```python
from build123d import *

# Parameters (mm, degrees)
SKETCH_W         = 93.98
SKETCH_H         = 98.425
SKETCH_R         = 2.2225
PAD_DEPTH        = 8.89
SKETCH001_W      = 44.45
SKETCH001_H      = 74.93
POCKET_DEPTH     = 2.286
SKETCH002_R      = 3.4925
PAD001_DEPTH     = 6.147
POCKET001_DEPTH  = 98.426
CHAMFER_SIZE     = 3.81
CHAMFER001_SIZE2 = 77.1906
CHAMFER001_SIZE  = 19.0246
CHAMFER002_SIZE  = 2.54


with BuildPart() as part:
    # Sketch → Pad (new body)
    with BuildSketch(Plane.XY):
        with Locations((0, 49.2125)):
            Rectangle(SKETCH_W, SKETCH_H)
        with Locations((37.5, 86.811)):
            Circle(SKETCH_R, mode=Mode.SUBTRACT)
        with Locations((-37.5, 86.811)):
            Circle(SKETCH_R, mode=Mode.SUBTRACT)
        with Locations((-37.5, 11.811)):
            Circle(SKETCH_R, mode=Mode.SUBTRACT)
        with Locations((37.5, 11.811)):
            Circle(SKETCH_R, mode=Mode.SUBTRACT)
    extrude(amount=PAD_DEPTH)

    # Sketch001 → Pocket (cut)
    with BuildSketch(Plane.XY):
        with Locations((0, 37.465)):
            Rectangle(SKETCH001_W, SKETCH001_H)
    extrude(amount=POCKET_DEPTH, mode=Mode.SUBTRACT)

    # Sketch002 → Pad001 (join)
    with BuildSketch(Plane.XZ):
        Polygon((-19.05, 8.89), (-19.05, 27.94), (19.05, 27.94), (19.05, 8.89), (46.99, 8.89), (46.99, 0), (85.572552, 0), (66.7766, -28.194), (-70.5866, -28.194), (-45.863996, 8.89), align=None)
        with Locations((0, -10.1346)):
            Circle(SKETCH002_R, mode=Mode.SUBTRACT)
    extrude(amount=PAD001_DEPTH)

    # Sketch003 → Pocket001 (cut, through all)
    with BuildSketch(Plane.XZ):
        Polygon((-45.863996, 8.89), (-45.863996, 18.360811), (-55.502193, 18.360811), (-55.502193, -5.567332), align=None)
    extrude(amount=-POCKET001_DEPTH, mode=Mode.SUBTRACT)

    # Chamfer
    chamfer_edges = [part.edges().sort_by_distance(p)[0] for p in [
        (-70.5866, -3.0735, -28.194),
        (85.572552, -3.0735, 0),
    ]]
    chamfer(chamfer_edges, length=CHAMFER_SIZE)

    # Chamfer001
    chamfer001_edges = [part.edges().sort_by_distance(p)[0] for p in [
        (0, 0, 8.89),
    ]]
    chamfer001_side = part.faces().sort_by_distance((0, 0, 18.415))[0]
    chamfer(chamfer001_edges, length=CHAMFER001_SIZE, length2=CHAMFER001_SIZE2, reference=chamfer001_side)

    # Chamfer002
    chamfer002_edges = [part.edges().sort_by_distance(p)[0] for p in [
        (-19.05, 38.5953, 8.89),
        (-19.05, -3.0735, 8.89),
        (-46.99, 98.425, 3.600495),
        (46.99, 98.425, 4.445),
        (19.05, -3.0735, 8.89),
        (19.05, 38.5953, 8.89),
        (19.05, -3.0735, 27.94),
        (-19.05, -3.0735, 27.94),
        (46.99, 46.139, 8.89),
        (46.99, -3.0735, 0),
    ]]
    chamfer(chamfer002_edges, length=CHAMFER002_SIZE)


solid = part.part
```
Source: CAD feature listing. Evaluate the final solid. Frame: model axes, mm. A direction names the side the tool comes from. Round coordinates to 2 decimals unless told otherwise and drop trailing zeros. Loops run counter-clockwise (first coordinate to the right, second up) from the corner with the lowest first, then second, coordinate; pieces in that order, holes last. Notation, with made-up numbers: M 5.25,9 L 59.25,9 A19 cw 59.25,20 Z; hole C -26,71.25 d6. An arc over 180 degrees is marked long. Use a Markdown table: item, result. Add a question column.
1. Cut plane B-B, the plane x = 0. Output: boundary loops of the cut face in (y, z) (3 decimals).
2. Contact query for flat-ended pins moving along their axis: pin 1 (3 mm diameter, centred on y = 33.5, z = 16, fed in from +X); pin 2 (1 mm diameter, centred on x = -9, y = 50.5, fed in from +Z); pin 3 (7 mm diameter, centred on x = -37.5, y = 11.811, fed in from -Z); pin 4 (2.5 mm diameter, centred on x = -37.5, y = 86.811, fed in from +Z). Output: stop coordinate, or through.
3. Pull-direction query (X, two-part tool) for faces 6 (the flat face through (19.05, 23, 17)), 7 (the flat face through (9, -6.147, -6)), 8 (the cylindrical face through (-39.264, 10.459, 4.383)); classes: +X half, -X half, draft (parallel to the pull), parting line (faces both ways), or undercut.
4. Cut plane A-A, the plane x = -37.5. Output: boundary loops of the cut face in (y, z) (1 decimal).
5. Set-up query: faces 1 (the flat face through (65, -3, 0)), 2 (the flat face through (-1, 82, 8.89)), 3 (the flat face through (75.235, -3.03, -15.507)), 4 (the flat face through (0, 38, 2.286)), 5 (the flat face through (-19.05, 23, 17)). Return all of +Z, -Z, +X, -X, +Y, -Y with unobstructed straight access to the full face (end or side cutting, diameter ignored); none if empty.
6. Cut plane D-D, the plane x = 59. Output: boundary loops of the cut face in (y, z), and give its area (3 significant figures).
7. Ray query, line 1 along Y through (x, z) = (-37.5, 3.25) (1 decimal); line 2 along X through (y, z) = (13, 2) (3 decimals); line 3 along Z through (x, y) = (0, -1). Return the intervals inside material, ascending. Write a range as [from, to].
8. Cut plane C-C, the plane y = 43. Output: boundary loops of the cut face in (x, z) (3 decimals).
Solution:
| question | item | result |
|---|---|---|
| 1 | outline | M -6.147,-28.194 L 0,-28.194 L 0,-13.627 L -6.147,-13.627 Z; M -6.147,-6.642 L 0,-6.642 L 0,2.286 L 74.93,2.286 L 74.93,0 L 98.425,0 L 98.425,8.89 L 77.191,8.89 L 0,27.915 L 0,27.94 L -6.147,27.94 Z |
| 2 | pin 1 | stops at x = 19.05 |
| 2 | pin 2 | stops at z = 15.59 |
| 2 | pin 3 | stops at z = 0 |
| 2 | pin 4 | passes through |
| 3 | face 6 | +X half |
| 3 | face 7 | draft |
| 3 | face 8 | undercut |
| 4 | outline | M -6.1,-28.2 L 0,-28.2 L 0,0 L 9.6,0 L 9.6,8.9 L -6.1,8.9 Z; M 14,0 L 84.6,0 L 84.6,8.9 L 14,8.9 Z; M 89,0 L 98.4,0 L 98.4,8.9 L 89,8.9 Z |
| 5 | face 1 | +Z, +X, +Y, -Y |
| 5 | face 2 | +Z, +Y |
| 5 | face 3 | -Z, +X, +Y, -Y |
| 5 | face 4 | -Z |
| 5 | face 5 | +Z, -X, +Y, -Y |
| 6 | outline | M -6.15,-28.19 L 0,-28.19 L 0,0 L -6.15,0 Z |
| 6 | area | 173 mm2 |
| 7 | line 1 | y = [-6.1, 9.6], [14, 84.6], [89, 98.4] |
| 7 | line 2 | x = [-46.99, -39.378], [-35.622, -22.225], [22.225, 35.622], [39.378, 46.99] |
| 7 | line 3 | z = [-28.19, -13.63], [-6.64, 27.94] |
| 8 | outline | M -46.99,0 L -22.225,0 L -22.225,2.286 L 22.225,2.286 L 22.225,0 L 46.99,0 L 46.99,6.35 L 44.45,8.89 L 21.59,8.89 L 19.05,11.43 L 19.05,17.317 L -19.05,17.317 L -19.05,11.43 L -21.59,8.89 L -45.864,8.89 L -46.99,7.201 Z |
